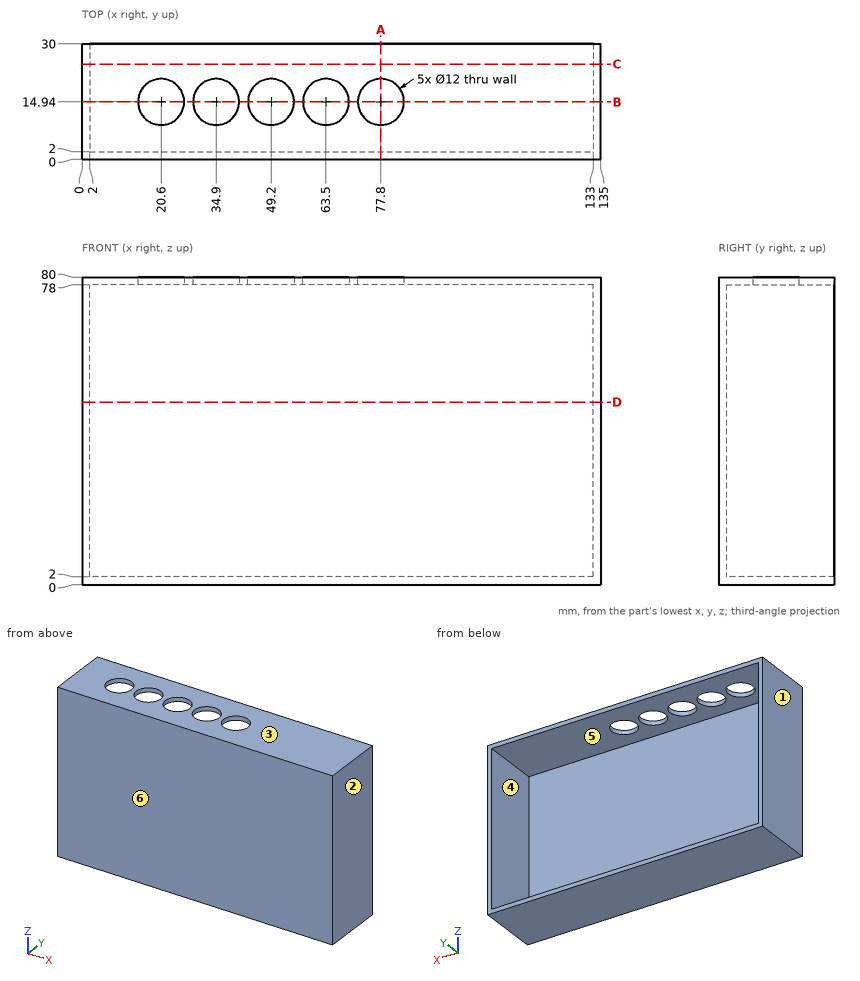
Source: three-view drawing plus pictorial views. Frame: mm from the lowest corner of the part. A direction names the side the tool comes from. Coordinates: 2 decimals unless noted, no trailing zeros. Loops run counter-clockwise (first coordinate to the right, second up) from the corner with the lowest first, then second, coordinate; pieces in that order, holes last. Notation, with made-up numbers: (60, 5) -> (66, 5) arc R23 ccw to (66, 44) -> close; hole circle Ø8 at (-29.5, 39.5). An arc over 180 degrees is marked (long way). Write each question's results on one line, items separated by ' | '. Start each with the question number.
Q1. Section C-C, the plane y = 24.75. Return the cut outline in (x, z).
Q2. Section A-A, the plane x = 77.8. Return the cut outline in (y, z).
Q3. Ray query, line 1 (X direction, y = 18.25, z = 44.5); line 2 (Z direction, x = 38, y = 25); line 3 (Y direction, x = 63.5, z = 78.7). Return the intervals inside material, ascending. Write a range as from..to.
Q4. Section D-D, the plane z = 47.5. Return the cut outline in (x, y), plus the area to 3 significant figures.
Q5. Pin query (flat end, axial travel): pin 1 (10 mm diameter, centred on x = 77, y = 11.5, fed in from +Z); pin 2 (4 mm diameter, centred on x = 16, z = 21.5, fed in from +Y). Return the tip coordinate at first contact, or that it passes through.
Q6. Section B-B, the plane y = 14.94. Return the cut outline in (x, z).
Q7. Pull-direction query (X, two-part tool) for the marked faces 1, 2, 3 and 4; classes: released by +X, released by -X, zero draft, split by the parting line, or undercut.
Q8. Reachability of the marked faces 5 and 6 from +Z, -Z, +X, -X, +Y, -Y: full face, straight path, thin tool, end or side. Return the list, or none.
Found:
1) outline: (0, 0) -> (135, 0) -> (135, 80) -> (0, 80) -> close; hole (2, 2) -> (133, 2) -> (133, 78) -> (2, 78) -> close
2) outline: (0, 0) -> (30, 0) -> (30, 2) -> (2, 2) -> (2, 78) -> (8.94, 78) -> (8.94, 80) -> (0, 80) -> close; (20.94, 78) -> (30, 78) -> (30, 80) -> (20.94, 80) -> close
3) line 1: 0..2, 133..135 | line 2: 0..2, 78..80 | line 3: 0..8.94, 20.94..30
4) outline: (0, 0) -> (135, 0) -> (135, 30) -> (133, 30) -> (133, 2) -> (2, 2) -> (2, 30) -> (0, 30) -> close | area: 382 mm2
5) pin 1: z = 80 | pin 2: y = 2
6) outline: (0, 0) -> (135, 0) -> (135, 80) -> (83.8, 80) -> (83.8, 78) -> (133, 78) -> (133, 2) -> (2, 2) -> (2, 78) -> (14.6, 78) -> (14.6, 80) -> (0, 80) -> close; (26.6, 78) -> (28.9, 78) -> (28.9, 80) -> (26.6, 80) -> close; (40.9, 78) -> (43.2, 78) -> (43.2, 80) -> (40.9, 80) -> close; (55.2, 78) -> (57.5, 78) -> (57.5, 80) -> (55.2, 80) -> close; (69.5, 78) -> (71.8, 78) -> (71.8, 80) -> (69.5, 80) -> close
7) face 1: released by -X | face 2: released by +X | face 3: zero draft | face 4: undercut
8) face 5: +Y | face 6: +Z, -Z, +X, -X, -Y
